from build123d import *

# Parameters (mm, degrees)
BOX004_W                 = 110
BOX004_H                 = 10
BOX004_DEPTH             = 10
ARRAY001_Y_COUNT         = 4
ARRAY001_Y_PITCH         = 20
ARRAY001_PLACEMENT_ANGLE = 90
BOX003_W                 = 110
BOX003_H                 = 10
BOX003_DEPTH             = 10
ARRAY_Y_COUNT            = 4
ARRAY_Y_PITCH            = 20
BOX002_W                 = 70
BOX002_H                 = 70
BOX002_DEPTH             = 110
BOX_W                    = 90
BOX_H                    = 90
BOX_DEPTH                = 150


with BuildPart() as obj1:
    # Box004 → Box004 (new body)
    with BuildSketch(Plane.XY):
        with Locations((55, 5)):
            Rectangle(BOX004_W, BOX004_H)
    extrude(amount=BOX004_DEPTH)

    # Array001 Y: obj1 ×4


with BuildPart() as obj1_1:
    add(obj1.part)
    with Locations(*[(0, i * ARRAY001_Y_PITCH, 0) for i in range(1, ARRAY001_Y_COUNT)]):
        add(obj1.part)


with BuildPart() as obj1_2:
    # Array001 placement: moved
    add(obj1_1.part.moved(Location((80, -10, 140))).rotate(Axis((80, -10, 140), (0, 0, 1)), ARRAY001_PLACEMENT_ANGLE))


with BuildPart() as barres:
    # Box003 → Box003 (new body)
    with BuildSketch(Plane.XY):
        with Locations((55, 5)):
            Rectangle(BOX003_W, BOX003_H)
    extrude(amount=BOX003_DEPTH)

    # Array Y: Barres ×4


with BuildPart() as barres_1:
    add(barres.part)
    with Locations(*[(0, i * ARRAY_Y_PITCH, 0) for i in range(1, ARRAY_Y_COUNT)]):
        add(barres.part)


with BuildPart() as barres_2:
    # Array placement: moved
    add(barres_1.part.moved(Location((-10, 10, 140))))

    # Fusion: union obj1
    add(obj1_2.part)


with BuildPart() as cub002:
    # Box002 → Box002 (new body)
    with BuildSketch(Plane(origin=(10, 10, 110), x_dir=(1, 0, 0), z_dir=(0, 0, 1))):
        with Locations((35, 35)):
            Rectangle(BOX002_W, BOX002_H)
    extrude(amount=BOX002_DEPTH)


with BuildPart() as obj2:
    # Box → Box (new body)
    with BuildSketch(Plane.XY):
        with Locations((45, 45)):
            Rectangle(BOX_W, BOX_H)
    extrude(amount=BOX_DEPTH)

    # Cut: cut Cub002
    add(cub002.part, mode=Mode.SUBTRACT)

    # Cut001: cut Barres
    add(barres_2.part, mode=Mode.SUBTRACT)


solid = obj2.part
Check sheet for the modelled part. Datum: model origin and axes. Units: mm. A direction names the side the tool comes from. Give positions to 0.01 mm unless a question says otherwise; leave off trailing zeros. Loops run counter-clockwise (first coordinate to the right, second up) from the corner with the lowest first, then second, coordinate; pieces in that order, holes last. Notation, with made-up numbers: M -30,-27.5 L 19,-27.5 A33 ccw 19,10.5 Z; hole C -27,-10 d4. An arc over 180 degrees is marked long. Use a Markdown table: item, result. Add a question column.
Q1. Sectioned sample at A-A, the plane z = 114.5. Record the cut outline in (x, y), then the cut area to 3 significant figures.
Q2. Mould release check, pull along Y, two halves, no side actions. Record for faces 4 (the flat face through (10, 45, 130)), 5 (the flat face through (80, 45, 130)), 6 (the flat face through (10, 85, 145)): pulls with the +Y half, pulls with the -Y half, needs draft (parallel to the pull), parting line crosses it, or undercut.
Q3. Tool access check on faces 1 (the flat face through (85, 15, 140)), 2 (the flat face through (85, 85, 150)), 3 (the flat face through (55, 85, 140)). Record the directions out of +Z, -Z, +X, -X, +Y, -Y that give a thin tool (end or side, any length) a straight path to the whole face; none if there is none.
Q4. Sectioned sample at B-B, the plane y = 42. Record the cut outline in (x, z), then the cut area to 3 significant figures.
Q5. Go/stop test with a flat-tipped pin: pin 1 (5 mm diameter, centred on x = 14, y = 87, fed in from +Z). Record where the tip stops, or that it passes through.
Q6. Sectioned sample at D-D, the plane x = 82.5. Record the cut outline in (y, z).
Q7. Scan lines: line 1 along Y through (x, z) = (26, 142.5); line 2 along Z through (x, y) = (65, 11). Record each from-to range of solid material in increasing order. Write a range as [from, to].
Verdict:
| question | item | result |
|---|---|---|
| 1 | outline | M 0,0 L 90,0 L 90,90 L 0,90 Z; hole M 10,10 L 80,10 L 80,80 L 10,80 Z |
| 1 | area | 3,200 mm^2 |
| 2 | face 4 | undercut |
| 2 | face 5 | undercut |
| 2 | face 6 | needs draft |
| 3 | face 1 | +Z, +X, -X |
| 3 | face 2 | +Z, +X, -X, +Y, -Y |
| 3 | face 3 | +Z, +Y, -Y |
| 4 | outline | M 0,0 L 90,0 L 90,150 L 80,150 L 80,110 L 10,110 L 10,150 L 0,150 Z |
| 4 | area | 10,700 mm^2 |
| 5 | pin 1 | z = 140 |
| 6 | outline | M 0,0 L 90,0 L 90,150 L 80,150 L 80,140 L 70,140 L 70,150 L 60,150 L 60,140 L 50,140 L 50,150 L 40,150 L 40,140 L 30,140 L 30,150 L 20,150 L 20,140 L 10,140 L 10,150 L 0,150 Z |
| 7 | line 1 | [0, 10], [80, 90] |
| 7 | line 2 | [0, 110] |
